from build123d import *

# Parameters (mm, degrees)
ROTATION1_ANGLE                      = 180
SCHNITT_LINEAR_AUSTRAGEN2_DEPTH      = 92.33454987
SCHNITT_LINEAR_AUSTRAGEN2_DEPTH_BACK = 90
SCHNITT_LINEAR_AUSTRAGEN3_DEPTH      = 92.33454987
SCHNITT_LINEAR_AUSTRAGEN3_DEPTH_BACK = 90
SKIZZE8_W                            = 10
SKIZZE8_H                            = 5
AUFSATZ_LINEAR_AUSTRAGEN2_DEPTH      = 90
SKIZZE9_W                            = 10
SKIZZE9_H                            = 5
AUFSATZ_LINEAR_AUSTRAGEN3_DEPTH      = 90
SKIZZE14_R                           = 2
SCHNITT_LINEAR_AUSTRAGEN7_DEPTH      = 93.258379674
SKIZZE16_R                           = 1
SCHNITT_LINEAR_AUSTRAGEN8_DEPTH      = 93.717898057
SKIZZE18_R                           = 4
SCHNITT_LINEAR_AUSTRAGEN9_DEPTH      = 5
SKIZZE20_W                           = 21.700648505
SKIZZE20_H                           = 2
SCHNITT_LINEAR_AUSTRAGEN10_DEPTH     = 93.717898057


with BuildPart() as part:
    # Skizze3 → Rotation1 (revolve)
    with BuildSketch(Plane.XY):
        Polygon((0, 0), (-11, 0), (-11, 90), (-6, 90), (-6, 10), (0, 10), align=None)
    revolve(axis=Axis((0, 0, 0), (0, 1, 0)), revolution_arc=ROTATION1_ANGLE)

    # Skizze6 → Schnitt-Linear austragen2 (cut, two sides: drawn at the far end of the back side and taken through both)
    with BuildSketch(Plane(origin=(0, 90, 0), x_dir=(1, 0, 0), z_dir=(0, 1, 0)).offset(-SCHNITT_LINEAR_AUSTRAGEN2_DEPTH_BACK)):
        Polygon((-9.380624863, -62.0642209), (-9.380624863, -5.744900102), (-9.380624863, 0), (-9.380624863, 56.319320799), (-122.01926646, 56.319320799), (-122.01926646, -62.0642209), align=None)
    extrude(amount=SCHNITT_LINEAR_AUSTRAGEN2_DEPTH + SCHNITT_LINEAR_AUSTRAGEN2_DEPTH_BACK, mode=Mode.SUBTRACT)

    # Skizze7 → Schnitt-Linear austragen3 (cut, two sides: drawn at the far end of the back side and taken through both)
    with BuildSketch(Plane.XZ.offset(-SCHNITT_LINEAR_AUSTRAGEN3_DEPTH_BACK)):
        Polygon((9.380624863, 59.241313346), (9.380624863, 5.744900102), (9.380624863, 0), (9.380624863, -53.496413245), (116.373451353, -53.496413245), (116.373451353, 59.241313346), align=None)
    extrude(amount=SCHNITT_LINEAR_AUSTRAGEN3_DEPTH + SCHNITT_LINEAR_AUSTRAGEN3_DEPTH_BACK, mode=Mode.SUBTRACT)

    # Skizze8 → Aufsatz-Linear austragen2 (add)
    with BuildSketch(Plane(origin=(0, 90, 0), x_dir=(1, 0, 0), z_dir=(0, 1, 0))):
        with Locations((-14.380624863, -2.5)):
            Rectangle(SKIZZE8_W, SKIZZE8_H)
    extrude(amount=-AUFSATZ_LINEAR_AUSTRAGEN2_DEPTH)

    # Skizze9 → Aufsatz-Linear austragen3 (add)
    with BuildSketch(Plane(origin=(0, 90, 0), x_dir=(1, 0, 0), z_dir=(0, 1, 0))):
        with Locations((14.380624863, -2.5)):
            Rectangle(SKIZZE9_W, SKIZZE9_H)
    extrude(amount=-AUFSATZ_LINEAR_AUSTRAGEN3_DEPTH)

    # Skizze14 → Schnitt-Linear austragen7 (cut, through all)
    with BuildSketch(Plane.XY.offset(5)):
        with Locations((-14.380624863, 80)):
            Circle(SKIZZE14_R)
        with Locations((-14.380624863, 10)):
            Circle(SKIZZE14_R)
        with Locations((14.380624863, 10)):
            Circle(SKIZZE14_R)
        with Locations((14.380624863, 80)):
            Circle(SKIZZE14_R)
    extrude(amount=-SCHNITT_LINEAR_AUSTRAGEN7_DEPTH, mode=Mode.SUBTRACT)

    # Skizze16 → Schnitt-Linear austragen8 (cut, through all)
    with BuildSketch(Plane.XZ):
        Circle(SKIZZE16_R)
    extrude(amount=-SCHNITT_LINEAR_AUSTRAGEN8_DEPTH, mode=Mode.SUBTRACT)

    # Skizze18 → Schnitt-Linear austragen9 (cut)
    with BuildSketch(Plane.XZ):
        Circle(SKIZZE18_R)
    extrude(amount=-SCHNITT_LINEAR_AUSTRAGEN9_DEPTH, mode=Mode.SUBTRACT)

    # Skizze20 → Schnitt-Linear austragen10 (cut, through all)
    with BuildSketch(Plane(origin=(0, 90, 0), x_dir=(1, 0, 0), z_dir=(0, 1, 0))):
        with Locations((-0.450220923, -10)):
            Rectangle(SKIZZE20_W, SKIZZE20_H)
    extrude(amount=-SCHNITT_LINEAR_AUSTRAGEN10_DEPTH, mode=Mode.SUBTRACT)


solid = part.part
Work out the finished part from the listing and answer in its coordinate system (mm). A direction names the side the tool comes from. Round coordinates to 2 decimals unless told otherwise and drop trailing zeros. Write each loop counter-clockwise with the first axis right and the second up, starting at its lowest first coordinate (ties: lowest second). Pieces come first, ordered by that corner, then holes. Notation, with made-up numbers: M 61,13 L 96,13 A31 ccw 96,50 Z; hole C -5,19 d10. An arc over 180 degrees is marked long. Use a Markdown table: item, result.
1) The part is cut by section A-A on y = 80. Give the vertices of the cut face in (x, z).
Taken from the geometry:
| item | result |
|---|---|
| outline | M -19.38,0 L -16.38,0 L -16.38,5 L -19.38,5 Z; M -12.38,0 L -6,0 A6 cw 6,0 L 12.38,0 L 12.38,5 L 9.38,5 L 9.38,5.74 A11 ccw 6.32,9 L -6.32,9 A11 ccw -9.38,5.74 L -9.38,5 L -12.38,5 Z; M 16.38,0 L 19.38,0 L 19.38,5 L 16.38,5 Z |
2) The part is cut by section C-C on z = 2.25. Give the vertices of the cut face in (x, y).
Taken from the geometry:
| item | result |
|---|---|
| outline | M -19.38,0 L -3.31,0 L -3.31,5 L 3.31,5 L 3.31,0 L 19.38,0 L 19.38,90 L 5.56,90 L 5.56,10 L -5.56,10 L -5.56,90 L -19.38,90 Z; hole C -14.38,10 d4; hole C -14.38,80 d4; hole C 14.38,10 d4; hole C 14.38,80 d4 |
3) The part is cut by section B-B on y = 39. Give the vertices of the cut face in (x, z).
Taken from the geometry:
| item | result |
|---|---|
| outline | M -19.38,0 L -6,0 A6 cw 6,0 L 19.38,0 L 19.38,5 L 9.38,5 L 9.38,5.74 A11 ccw 6.32,9 L -6.32,9 A11 ccw -9.38,5.74 L -9.38,5 L -19.38,5 Z |
4) The part is cut by section D-D on x = -14. Give the vertices of the cut face in (y, z), plus the area to 3 significant figures.
Taken from the geometry:
| item | result |
|---|---|
| outline | M 0,0 L 8.04,0 L 8.04,5 L 0,5 Z; M 11.96,0 L 78.04,0 L 78.04,5 L 11.96,5 Z; M 81.96,0 L 90,0 L 90,5 L 81.96,5 Z |
| area | 411 mm2 |
5) Determine the mould class of faces 5 (the face through (15.456, 11.686, 2.535)), 6 (the face through (-14, 46, 5)), 7 (the face through (-8.04, 45.63, 7.51)), 8 (the face through (14.12, 81.983, 2.535)) for opening direction X: pulls with the +X half, pulls with the -X half, needs draft (parallel to the pull), parting line crosses it, or undercut.
Taken from the geometry:
| item | result |
|---|---|
| face 5 | undercut |
| face 6 | needs draft |
| face 7 | pulls with the -X half |
| face 8 | undercut |
6) Flat-ended cylindrical pins translate along their axes: pin 1 (2 mm diameter, centred on x = 0, z = 2.5, fed in from -Y); pin 2 (5 mm diameter, centred on x = -14.5, y = 33, fed in from +Z); pin 3 (0.6 mm diameter, centred on y = 64.5, z = 5.5, fed in from +X); pin 4 (3.5 mm diameter, centred on x = 14.38, y = 80, fed in from -Z). Find the tip coordinate at first contact, or state that the pin passes through.
Taken from the geometry:
| item | result |
|---|---|
| pin 1 | stops at y = 5 |
| pin 2 | stops at z = 5 |
| pin 3 | stops at x = 9.38 |
| pin 4 | passes through |
7) Which of the six approach directions +Z, -Z, +X, -X, +Y, -Y give full straight-line access (tool end or side, diameter ignored) to faces 1 (the face through (0, 5, 2)), 2 (the face through (0, 49, 6)), 3 (the face through (14, 46, 5)), 4 (the face through (0, 7, 1))?
Taken from the geometry:
| item | result |
|---|---|
| face 1 | -Z, -Y |
| face 2 | -Z, +Y |
| face 3 | +Z, +X, +Y, -Y |
| face 4 | -Z, +Y, -Y |
8) Consider line 1 (Y direction, x = -15, z = 1.25); line 2 (Z direction, x = -15.5, y = 36); line 3 (Z direction, x = 0, y = 76). Determine where each line is inside the solid, lowest interval first. Write a range as [from, to].
Taken from the geometry:
| item | result |
|---|---|
| line 1 | y = [0, 8.1], [11.9, 78.1], [81.9, 90] |
| line 2 | z = [0, 5] |
| line 3 | z = [6, 9] |
